```python
from build123d import *

# Parameters (mm, degrees)
BOSS_EXTRUDE1_DEPTH      = 34
BOSS_EXTRUDE1_DEPTH_BACK = 30
SKETCH2_W                = 60
SKETCH2_H                = 44
CUT_EXTRUDE1_DEPTH       = 36.4
CUT_EXTRUDE2_DEPTH       = 1.6
BOSS_EXTRUDE2_DEPTH      = 1.5
CHAMFER1_SIZE            = 2
CUT_EXTRUDE3_REACH       = 70.207
SKETCH8_W                = 20
SKETCH8_H                = 12
CUT_EXTRUDE4_DEPTH       = 1.5
BOSS_EXTRUDE3_REACH      = 86.994
CUT_EXTRUDE7_REACH       = 61.23
SKETCH12_W               = 52
SKETCH12_H               = 18.301043111
CHAMFER2_SIZE            = 2
BOSS_EXTRUDE4_DEPTH      = 60
BOSS_EXTRUDE5_DEPTH      = 2


with BuildPart() as part:
    # Sketch1 → Boss-Extrude1 (new, two sides: drawn at the far end of the back side and taken through both)
    with BuildSketch(Plane(origin=(0, 0, 0), x_dir=(0, 0, -1), z_dir=(1, 0, 0)).offset(-BOSS_EXTRUDE1_DEPTH_BACK)):
        Polygon((0, 38), (0, 0), (44, 0), (44, 9.717345174), (10.294044503, 38), align=None)
    extrude(amount=BOSS_EXTRUDE1_DEPTH + BOSS_EXTRUDE1_DEPTH_BACK)

    # Sketch2 → Cut-Extrude1 (cut)
    with BuildSketch(Plane(origin=(0, 38, 0), x_dir=(1, 0, 0), z_dir=(0, 1, 0))):
        with Locations((2, 22)):
            Rectangle(SKETCH2_W, SKETCH2_H)
    extrude(amount=-CUT_EXTRUDE1_DEPTH, mode=Mode.SUBTRACT)

    # Sketch5 → Cut-Extrude2 (cut)
    with BuildSketch(Plane.XZ):
        Polygon((-20, -12), (20, -12), (34, -3.917096231), (34, 0), (-30, 0), (-30, -6.226497308), align=None)
    extrude(amount=-CUT_EXTRUDE2_DEPTH, mode=Mode.SUBTRACT)

    # Sketch6 → Boss-Extrude2 (add)
    with BuildSketch(Plane.XZ):
        Polygon((-30, 0), (-30, -8.535898385), (-20.535898385, -14), (20.535898385, -14), (34, -6.226497308), (34, 0), align=None)
    extrude(amount=BOSS_EXTRUDE2_DEPTH)

    # Chamfer1
    # the kernel refuses this chamfer: 2 mm, written as the material it adds along each edge
    with BuildSketch(Plane(origin=(16.081612789, 0, -16.571682988), x_dir=(0.4998109584556485, 0.027495876610586344, -0.8656979742248803), z_dir=(0.8660254037844386, 0, 0.5000000000000001))) as chamfer1_piece_1_section:
        Polygon((CHAMFER1_SIZE * 0.999621916911, -CHAMFER1_SIZE * 0.0274958766106), (-CHAMFER1_SIZE * 0.0274958766106, -CHAMFER1_SIZE * 0.999621916911), (0, 0), align=None)
    chamfer1_piece_1 = extrude(amount=25.833737336, mode=Mode.PRIVATE)
    chamfer1_piece_1 = split(chamfer1_piece_1, bisect_by=Plane(origin=(34, -0.590941393, -10.495986371), z_dir=(-1, 0, 0)), keep=Keep.TOP, mode=Mode.PRIVATE)
    chamfer1_piece_1 = split(chamfer1_piece_1, bisect_by=Plane(origin=(27.930870364, -0.590941393, -14), z_dir=(0, 0, 1)), keep=Keep.TOP, mode=Mode.PRIVATE)
    chamfer1_piece_1 = split(chamfer1_piece_1, bisect_by=Plane(origin=(27.930870364, -1.5, -10.495986371), z_dir=(0, 1, 0)), keep=Keep.TOP, mode=Mode.PRIVATE)
    add(chamfer1_piece_1)
    with BuildSketch(Plane(origin=(-34.454285596, 0, -5.964215397), x_dir=(-0.4998109584556484, 0.027495876610586348, -0.8656979742248804), z_dir=(0.8660254037844387, 0, -0.5))) as chamfer1_piece_2_section:
        Polygon((CHAMFER1_SIZE * 0.999621916911, -CHAMFER1_SIZE * 0.0274958766106), (-CHAMFER1_SIZE * 0.0274958766106, -CHAMFER1_SIZE * 0.999621916911), (0, 0), align=None)
    chamfer1_piece_2 = extrude(amount=21.214935182, mode=Mode.PRIVATE)
    chamfer1_piece_2 = split(chamfer1_piece_2, bisect_by=Plane(origin=(-30, -0.598869914, -11.638934736), z_dir=(1, 0, 0)), keep=Keep.TOP, mode=Mode.PRIVATE)
    chamfer1_piece_2 = split(chamfer1_piece_2, bisect_by=Plane(origin=(-25.910515002, -1.5, -11.638934736), z_dir=(0, 1, 0)), keep=Keep.TOP, mode=Mode.PRIVATE)
    chamfer1_piece_2 = split(chamfer1_piece_2, bisect_by=Plane(origin=(-25.910515002, -0.598869914, -14), z_dir=(0, 0, 1)), keep=Keep.TOP, mode=Mode.PRIVATE)
    add(chamfer1_piece_2)
    with BuildSketch(Plane(origin=(-25.679264361, 0, -14), x_dir=(0, 0.027495876610586424, -0.9996219169112968), z_dir=(1, 0, 0))) as chamfer1_piece_3_section:
        Polygon((CHAMFER1_SIZE * 0.999621916911, -CHAMFER1_SIZE * 0.0274958766106), (-CHAMFER1_SIZE * 0.0274958766106, -CHAMFER1_SIZE * 0.999621916911), (0, 0), align=None)
    chamfer1_piece_3 = extrude(amount=51.358528722, mode=Mode.PRIVATE)
    chamfer1_piece_3 = split(chamfer1_piece_3, bisect_by=Plane(origin=(4.838764491, -0.58360414, -23.062744479), z_dir=(-0.5000000000000001, 0, 0.8660254037844386)), keep=Keep.TOP, mode=Mode.PRIVATE)
    chamfer1_piece_3 = split(chamfer1_piece_3, bisect_by=Plane(origin=(0, -1.5, -14.681758534), z_dir=(0, 1, 0)), keep=Keep.TOP, mode=Mode.PRIVATE)
    chamfer1_piece_3 = split(chamfer1_piece_3, bisect_by=Plane(origin=(-4.838764491, -0.58360414, -23.062744479), z_dir=(0.5, 0, 0.8660254037844387)), keep=Keep.TOP, mode=Mode.PRIVATE)
    add(chamfer1_piece_3)
    with BuildSketch(Plane(origin=(16.081612789, 0, -16.571682988), x_dir=(0.4998109584556485, 0.027495876610586344, -0.8656979742248803), z_dir=(0.8660254037844386, 0, 0.5000000000000001))) as chamfer1_piece_4a_section:
        Polygon((CHAMFER1_SIZE * 0.999621916911, -CHAMFER1_SIZE * 0.0274958766106), (-CHAMFER1_SIZE * 0.0274958766106, -CHAMFER1_SIZE * 0.999621916911), (0, 0), align=None)
    chamfer1_piece_4a = extrude(amount=25.833737336, mode=Mode.PRIVATE)
    chamfer1_piece_4a = split(chamfer1_piece_4a, bisect_by=Plane(origin=(19.272748758, -0.548768343, -14), z_dir=(0, 0, -1)), keep=Keep.TOP, mode=Mode.PRIVATE)
    chamfer1_piece_4a = split(chamfer1_piece_4a, bisect_by=Plane(origin=(19.272748758, -1.5, -15.619778524), z_dir=(0, 1, 0)), keep=Keep.TOP, mode=Mode.PRIVATE)
    with BuildSketch(Plane(origin=(-25.679264361, 0, -14), x_dir=(0, 0.027495876610586424, -0.9996219169112968), z_dir=(1, 0, 0))) as chamfer1_piece_4b_section:
        Polygon((CHAMFER1_SIZE * 0.999621916911, -CHAMFER1_SIZE * 0.0274958766106), (-CHAMFER1_SIZE * 0.0274958766106, -CHAMFER1_SIZE * 0.999621916911), (0, 0), align=None)
    chamfer1_piece_4b = extrude(amount=51.358528722, mode=Mode.PRIVATE)
    chamfer1_piece_4b = split(chamfer1_piece_4b, bisect_by=Plane(origin=(21.62981805, -0.548768343, -13.368425187), z_dir=(0.5000000000000001, 0, -0.8660254037844386)), keep=Keep.TOP, mode=Mode.PRIVATE)
    chamfer1_piece_4b = split(chamfer1_piece_4b, bisect_by=Plane(origin=(22.439707312, -1.5, -14.771194537), z_dir=(0, 1, 0)), keep=Keep.TOP, mode=Mode.PRIVATE)
    chamfer1_piece_4 = chamfer1_piece_4a & chamfer1_piece_4b
    add(chamfer1_piece_4)
    with BuildSketch(Plane(origin=(-25.679264361, 0, -14), x_dir=(0, 0.027495876610586424, -0.9996219169112968), z_dir=(1, 0, 0))) as chamfer1_piece_5a_section:
        Polygon((CHAMFER1_SIZE * 0.999621916911, -CHAMFER1_SIZE * 0.0274958766106), (-CHAMFER1_SIZE * 0.0274958766106, -CHAMFER1_SIZE * 0.999621916911), (0, 0), align=None)
    chamfer1_piece_5a = extrude(amount=51.358528722, mode=Mode.PRIVATE)
    chamfer1_piece_5a = split(chamfer1_piece_5a, bisect_by=Plane(origin=(-22.439707312, -1.5, -14.771194537), z_dir=(0, 1, 0)), keep=Keep.TOP, mode=Mode.PRIVATE)
    chamfer1_piece_5a = split(chamfer1_piece_5a, bisect_by=Plane(origin=(-21.62981805, -0.548768343, -13.368425187), z_dir=(-0.5, 0, -0.8660254037844387)), keep=Keep.TOP, mode=Mode.PRIVATE)
    with BuildSketch(Plane(origin=(-34.454285596, 0, -5.964215397), x_dir=(-0.4998109584556484, 0.027495876610586348, -0.8656979742248804), z_dir=(0.8660254037844387, 0, -0.5))) as chamfer1_piece_5b_section:
        Polygon((CHAMFER1_SIZE * 0.999621916911, -CHAMFER1_SIZE * 0.0274958766106), (-CHAMFER1_SIZE * 0.0274958766106, -CHAMFER1_SIZE * 0.999621916911), (0, 0), align=None)
    chamfer1_piece_5b = extrude(amount=21.214935182, mode=Mode.PRIVATE)
    chamfer1_piece_5b = split(chamfer1_piece_5b, bisect_by=Plane(origin=(-19.272748758, -1.5, -15.619778524), z_dir=(0, 1, 0)), keep=Keep.TOP, mode=Mode.PRIVATE)
    chamfer1_piece_5b = split(chamfer1_piece_5b, bisect_by=Plane(origin=(-19.272748758, -0.548768343, -14), z_dir=(0, 0, -1)), keep=Keep.TOP, mode=Mode.PRIVATE)
    chamfer1_piece_5 = chamfer1_piece_5a & chamfer1_piece_5b
    add(chamfer1_piece_5)

    # Cut-Extrude3: up to this face of the body (flat: up to its plane)
    cut_extrude3_end = Plane(part.part.faces().sort_by_distance((2.35859889, 0, -29.378927014))[0])
    # Sketch7 → Cut-Extrude3 (cut, up to the picked face)
    with BuildSketch(Plane(origin=(0, 38, 0), x_dir=(1, 0, 0), z_dir=(0, 1, 0)), mode=Mode.PRIVATE) as cut_extrude3_sk1:
        Polygon((-30, 41.263838853), (-22.482459034, 44), (-30, 44), align=None)
    cut_extrude3_tool1 = split(extrude(cut_extrude3_sk1.sketch, amount=-CUT_EXTRUDE3_REACH, mode=Mode.PRIVATE), bisect_by=cut_extrude3_end, keep=Keep.BOTH, mode=Mode.PRIVATE)
    # Sketch7 → Cut-Extrude3 (cut, up to the picked face)
    with BuildSketch(Plane(origin=(0, 38, 0), x_dir=(1, 0, 0), z_dir=(0, 1, 0)), mode=Mode.PRIVATE) as cut_extrude3_sk2:
        Polygon((26.482459034, 44), (34, 41.263838853), (34, 44), align=None)
    cut_extrude3_tool2 = split(extrude(cut_extrude3_sk2.sketch, amount=-CUT_EXTRUDE3_REACH, mode=Mode.PRIVATE), bisect_by=cut_extrude3_end, keep=Keep.BOTH, mode=Mode.PRIVATE)
    add(cut_extrude3_tool1.solids().sort_by(Axis((-27.494153, 38, -43.087946), (0, -1, 0)))[0], mode=Mode.SUBTRACT)
    add(cut_extrude3_tool2.solids().sort_by(Axis((31.494153, 38, -43.087946), (0, -1, 0)))[0], mode=Mode.SUBTRACT)

    # Sketch8 → Cut-Extrude4 (cut)
    with BuildSketch(Plane(origin=(0, 0, 0), x_dir=(1, 0, 0), z_dir=(0, 1, 0))):
        with Locations((0, 6)):
            Rectangle(SKETCH8_W, SKETCH8_H)
    extrude(amount=-CUT_EXTRUDE4_DEPTH, mode=Mode.SUBTRACT)

    # Boss-Extrude3: up to this face of the body (flat: up to its plane)
    boss_extrude3_end = Plane(part.part.faces().sort_by_distance((32, 16.245464339, -17.024050876))[0])
    # Sketch11 → Boss-Extrude3 (add, up to the picked face)
    with BuildSketch(Plane(origin=(-28, 0, 0), x_dir=(0, 0, -1), z_dir=(1, 0, 0)), mode=Mode.PRIVATE) as boss_extrude3_sk1:
        Polygon((15.937131869, 17.6), (30.23817498, 5.6), (30.23817498, 1.6), (11.937131869, 1.6), (11.937131869, 17.6), align=None)
    boss_extrude3_tool1 = split(extrude(boss_extrude3_sk1.sketch, amount=BOSS_EXTRUDE3_REACH, mode=Mode.PRIVATE), bisect_by=boss_extrude3_end, keep=Keep.BOTH, mode=Mode.PRIVATE)
    add(boss_extrude3_tool1.solids().sort_by(Axis((-28, 7.941992, -19.27068), (1, 0, 0)))[0])

    # Cut-Extrude7: up to this face of the body (flat: up to its plane)
    cut_extrude7_end = Plane(part.part.faces().sort_by_distance((2, 1.6, -37.034599694))[0])
    # Sketch12 → Cut-Extrude7 (cut, up to the picked face)
    with BuildSketch(Plane(origin=(0, 17.6, 0), x_dir=(1, 0, 0), z_dir=(0, 1, 0)), mode=Mode.PRIVATE) as cut_extrude7_sk1:
        with Locations((2, 21.087653425)):
            Rectangle(SKETCH12_W, SKETCH12_H)
    cut_extrude7_tool1 = split(extrude(cut_extrude7_sk1.sketch, amount=-CUT_EXTRUDE7_REACH, mode=Mode.PRIVATE), bisect_by=cut_extrude7_end, keep=Keep.BOTH, mode=Mode.PRIVATE)
    add(cut_extrude7_tool1.solids().sort_by(Axis((2, 17.6, -21.087653), (0, -1, 0)))[0], mode=Mode.SUBTRACT)

    # Chamfer2
    chamfer2_edges = [part.edges().sort_by_distance(p)[0] for p in [
        (10, -0.75, 0),
        (-10, -0.75, 0),
    ]]
    chamfer(chamfer2_edges, length=CHAMFER2_SIZE)

    # Sketch14 → Boss-Extrude4 (add)
    with BuildSketch(Plane(origin=(-28, 0, 0), x_dir=(0, 0, -1), z_dir=(1, 0, 0))):
        Polygon((41.991779322, 3.6), (41.991779322, 1.6), (39.991779322, 1.6), align=None)
    extrude(amount=BOSS_EXTRUDE4_DEPTH)

    # Sketch15 → Boss-Extrude5 (add)
    with BuildSketch(Plane(origin=(0, 1.6, 0), x_dir=(1, 0, 0), z_dir=(0, 1, 0))):
        Polygon((-28, 41.991779322), (32, 41.991779322), (26.482459034, 44), (-22.482459034, 44), align=None)
    extrude(amount=BOSS_EXTRUDE5_DEPTH)


solid = part.part
```
Here's how the part is built. I have some questions about the finished solid (model axes, mm). A direction names the side the tool comes from. Round coordinates to 2 decimals unless told otherwise and drop trailing zeros. Order: outer loops, then holes, each group sorted by start corner. A loop starts at its lowest first (then second) coordinate and runs counter-clockwise, first axis right, second up. Notation, with made-up numbers: M 61.25,68 L 86.25,68 A14 ccw 86.25,76 Z; hole C 22.25,62 d1. An arc over 180 degrees is marked long. Answer as CSV lines item,"result".
Item 1: Imagine slicing it at B-B on x = 8.5. List the corners of the cut face in (y, z) for me.
From the geometry:
outline,"M -1.5,-14.5 L 0,-16 L 0,-44 L 3.6,-44 L 3.6,-41.99 L 1.6,-39.99 L 1.6,-12 L -1.5,-12 Z"
Item 2: Please list where these lines run through material, in increasing order: L1, parallel to X at y = 22, z = -3; L2, parallel to Y at x = 4.5, z = -24; L3, parallel to X at y = 2.5, z = -25. Write a range as [from, to].
From the geometry:
L1,"[-30, -28], [32, 34]"
L2,"[0, 1.6]"
L3,"[-30, -24], [28, 34]"
Item 3: We'd pull the mould along X, two halves only. Please class faces 6 (the flat face through (11, -1, -1)), 7 (the flat face through (-29, 38, -5)), 8 (the flat face through (27.445, -0.74, -11.466)): +X half, -X half, draft (parallel to the pull), parting line (faces both ways), or undercut.
From the geometry:
face 6,"undercut"
face 7,"draft"
face 8,"+X half"
Item 4: Imagine slicing it at C-C on z = -36. List the corners of the cut face in (x, y) for me.
From the geometry:
outline,"M -30,0 L 34,0 L 34,16.43 L 32,16.43 L 32,1.6 L -28,1.6 L -28,16.43 L -30,16.43 Z"
Item 5: Imagine slicing it at A-A on y = 21. List the corners of the cut face in (x, z) for me.
From the geometry:
outline,"M -30,-30.55 L -28,-30.55 L -28,0 L -30,0 Z; M 32,-30.55 L 34,-30.55 L 34,0 L 32,0 Z"
Item 6: Which directions (+Z, -Z, +X, -X, +Y, -Y) give clear straight access to the entire face, cutting with the end or side of a thin tool? Please do faces 1 (the flat face through (29.97, 11.68, -22.99)), 2 (the flat face through (32, 20, -16)), 3 (the flat face through (-10, -1, -7)), 4 (the flat face through (30, 17.6, -14)), 5 (the flat face through (-26, 9, -11.937)).
From the geometry:
face 1,"-Z, +Y"
face 2,"+Y"
face 3,"+Z, +Y, -Y"
face 4,"+Z, -Z, +Y"
face 5,"+Z, +Y"
Item 7: For pin 1 (0.6 mm diameter, centred on x = 11, z = -43, fed in from +Y); pin 2 (17.5 mm diameter, centred on x = 16.5, z = -29, fed in from -Y); pin 3 (1.2 mm diameter, centred on x = 31, y = 2.5, fed in from -Z); pin 4 (5 mm diameter, centred on x = -5.5, z = -9, fed in from +Y), each with a flat end and sliding along its axis, tell me the tip position at first contact or that it passes through.
From the geometry:
pin 1,"y = 3.6"
pin 2,"y = 0"
pin 3,"z = -42.57"
pin 4,"through"
Item 8: Imagine slicing it at D-D on y = 28.5. List the corners of the cut face in (x, z) for me.
From the geometry:
outline,"M -30,-21.62 L -28,-21.62 L -28,0 L -30,0 Z; M 32,-21.62 L 34,-21.62 L 34,0 L 32,0 Z"
